Here's how the part is built. I have some questions about the finished solid (model axes, mm). A direction names the side the tool comes from. Round coordinates to 2 decimals unless told otherwise and drop trailing zeros. Order: outer loops, then holes, each group sorted by start corner. A loop starts at its lowest first (then second) coordinate and runs counter-clockwise, first axis right, second up. Notation, with made-up numbers: (4.25, 44) -> (37.25, 44) arc R25 ccw to (37.25, 83) -> close; hole circle Ø7 at (54.5, -39). An arc over 180 degrees is marked (long way). Use a Markdown table: item, result. Add a question column.
(1) On a 3-axis mill with a long thin cutter (end or side, diameter ignored), from which of +Z, -Z, +X, -X, +Y, -Y can I reach the whole of each face in a straight line? I mean faces 5 (the face through (-10.478, 26, 3)), 6 (the face through (14, 16.828, 3)), 7 (the face through (-14.288, 0, 5)). Say none if no direction works.
(2) Thinking about a two-plate mould opening in X: for faces 1 (the face through (-7.938, 25, 5)), 2 (the face through (-16.828, 0, 3)), 3 (the face through (0, 35.878, 3)), 4 (the face through (0, 14.288, 4)), which applies, pulls with the +X half, pulls with the -X half, needs draft (parallel to the pull), parting line crosses it, or undercut?
(3) If I drill on probe 1 along Y at (x, z) = (1.5, 4); probe 2 along X at (y, z) = (19, 5); probe 3 along Y at (x, z) = (-6, 2.25), over which ranges is the centre line in solid material (lowest first)?
(4) I'm going to push flat-ended pins straight in: P1, Ø1.6, axis at y = 28, z = 4.5, coming from the -X side; P2, Ø1, axis at y = 24, z = 5, coming from the +X side; P3, Ø8, axis at x = -1, y = 23.5, coming from the +Z side (3 decimals). Where does each tip first touch, or does it pass through?
(5) I want a section at B-B, the plane z = 4.25. Please give me the cut outline in (x, y), then the cut area to 3 significant figures.
from build123d import *

# Parameters (mm, degrees)
F2_DEPTH = 3.175
F4_DEPTH = 6.35
F5_W     = 15.875
F5_H     = 2.54
F6_DEPTH = 3.175
F7_W     = 12.7
F7_H     = 2.54
F8_DEPTH = 25.4


with BuildPart() as f2:
    # F1 (on offset) → F2 (new body)
    with BuildSketch(Plane.XY):
        Polygon((-7.9375, 14.2875), (-14.2875, 14.2875), (-14.2875, -14.2875), (14.2875, -14.2875), (14.2875, 14.2875), (7.9375, 14.2875), (7.9375, 33.3375), (-7.9375, 33.3375), align=None)
    extrude(amount=F2_DEPTH)

    # F3 (on face) → F4 (join)
    with BuildSketch(Plane(origin=(0, 0, 0), x_dir=(1, 0, 0), z_dir=(0, 0, -1))):
        Polygon((16.8275, -16.8275), (16.8275, 16.8275), (-16.8275, 16.8275), (-16.8275, -16.8275), (-10.4775, -16.8275), (-10.4775, -35.8775), (10.4775, -35.8775), (10.4775, -16.8275), align=None)
        Polygon((-14.2875, 14.2875), (14.2875, 14.2875), (14.2875, -14.2875), (7.9375, -14.2875), (7.9375, -33.3375), (-7.9375, -33.3375), (-7.9375, -14.2875), (-14.2875, -14.2875), align=None, mode=Mode.SUBTRACT)
    extrude(amount=-F4_DEPTH)

    # F5 (on face) → F6 (join, through all)
    with BuildSketch(Plane.XY.offset(3.175)):
        with Locations((0, 15.5575)):
            Rectangle(F5_W, F5_H)
    extrude(amount=F6_DEPTH)

    # F7 (on face) → F8 (cut)
    with BuildSketch(Plane.XY.offset(3.175)):
        with Locations((0, 13.0175)):
            Rectangle(F7_W, F7_H)
    extrude(amount=-F8_DEPTH, mode=Mode.SUBTRACT)


solid = f2.part
Taken from the geometry:
| question | item | result |
|---|---|---|
| 1 | face 5 | +Z, -Z, -X, +Y |
| 1 | face 6 | +Z, -Z, +X, +Y |
| 1 | face 7 | +Z |
| 2 | face 1 | undercut |
| 2 | face 2 | pulls with the -X half |
| 2 | face 3 | needs draft |
| 2 | face 4 | undercut |
| 3 | probe 1 | y = -16.83 to -14.29, 14.29 to 16.83, 33.34 to 35.88 |
| 3 | probe 2 | x = -10.48 to -7.94, 7.94 to 10.48 |
| 3 | probe 3 | y = -16.83 to 11.75, 14.29 to 35.88 |
| 4 | P1 | stops at x = -10.48 |
| 4 | P2 | stops at x = 10.48 |
| 4 | P3 | stops at z = 3.175 |
| 5 | outline | (-16.83, -16.83) -> (16.83, -16.83) -> (16.83, 16.83) -> (10.48, 16.83) -> (10.48, 35.88) -> (-10.48, 35.88) -> (-10.48, 16.83) -> (-16.83, 16.83) -> close; hole (-14.29, -14.29) -> (14.29, -14.29) -> (14.29, 14.29) -> (-14.29, 14.29) -> close; hole (-7.94, 16.83) -> (7.94, 16.83) -> (7.94, 33.34) -> (-7.94, 33.34) -> close |
| 5 | area | 453 mm2 |
